from build123d import *

# Parameters (mm, degrees)
SALIENTE_EXTRUIR1_DEPTH  = 100
CROQUIS4_W               = 90
CROQUIS4_H               = 70
CORTAR_EXTRUIR1_DEPTH    = 44
SALIENTE_EXTRUIR2_DEPTH  = 19
SALIENTE_EXTRUIR4_START  = 19
SALIENTE_EXTRUIR4_DEPTH  = 19
SALIENTE_EXTRUIR7_DEPTH  = 13
SALIENTE_EXTRUIR28_START = 13
CROQUIS11_W              = 34
CROQUIS11_H              = 2.5
SALIENTE_EXTRUIR28_DEPTH = 13
CROQUIS13_W              = 28
CROQUIS13_H              = 6
SALIENTE_EXTRUIR10_DEPTH = 24
CROQUIS15_R              = 1.5
CORTAR_EXTRUIR2_DEPTH    = 5
CORTAR_EXTRUIR3_DEPTH    = 24
SALIENTE_EXTRUIR12_START = -28
SALIENTE_EXTRUIR12_DEPTH = 28
SALIENTE_EXTRUIR13_DEPTH = 52
SALIENTE_EXTRUIR14_DEPTH = 100
CORTAR_EXTRUIR4_DEPTH    = 24
SALIENTE_EXTRUIR15_DEPTH = 24
CORTAR_EXTRUIR7_DEPTH    = 90
SALIENTE_EXTRUIR27_DEPTH = 14
CORTAR_EXTRUIR12_DEPTH   = 90
CROQUIS41_R              = 2.6
CORTAR_EXTRUIR13_DEPTH   = 10
CROQUIS42_W              = 26
CROQUIS42_H              = 3.651340431
CORTAR_EXTRUIR14_DEPTH   = 121.043742028
CROQUIS37_W              = 5
CROQUIS37_H              = 25
CORTAR_EXTRUIR15_DEPTH   = 4
CROQUIS44_R              = 1.5
CORTAR_EXTRUIR16_DEPTH   = 4


with BuildPart() as part:
    # Croquis1 → Saliente-Extruir1 (new body)
    with BuildSketch(Plane(origin=(0, 0, 0), x_dir=(0, 0, -1), z_dir=(1, 0, 0))):
        with BuildLine():
            Line((50, 24), (50, 56))
            Line((50, 56), (-1.5, 56))
            Line((-1.5, 56), (-9.741455248, 56))
            ThreePointArc((-9.741455248, 56), (-16.048737738, 53.76003786), (-19.530405432, 48.043637519))
            Line((-19.530405432, 48.043637519), (-26.9291309, 12.604008733))
            Line((-26.9291309, 12.604008733), (-35.5, 0))
            Line((-35.5, 0), (-20, 0))
            Line((-20, 0), (-20, 14))
            ThreePointArc((-20, 14), (-17.071067812, 21.071067812), (-10, 24))
            Line((-10, 24), (50, 24))
        make_face()
    extrude(amount=SALIENTE_EXTRUIR1_DEPTH)

    # Croquis4 → Cortar-Extruir1 (cut, symmetric)
    with BuildSketch(Plane.XY):
        with Locations((50, 35)):
            Rectangle(CROQUIS4_W, CROQUIS4_H)
    extrude(amount=CORTAR_EXTRUIR1_DEPTH, both=True, mode=Mode.SUBTRACT)

    # Croquis5 → Saliente-Extruir2 (add)
    with BuildSketch(Plane(origin=(5, 0, 0), x_dir=(0, 0, -1), z_dir=(1, 0, 0))):
        with BuildLine():
            Line((-20, 0), (-20, 14))
            ThreePointArc((-20, 14), (-17.071067812, 21.071067812), (-10, 24))
            Line((-10, 24), (50, 24))
            Line((50, 24), (50, 26.5))
            Line((50, 26.5), (-10, 26.5))
            ThreePointArc((-10, 26.5), (-18.838834765, 22.838834765), (-22.5, 14))
            Line((-22.5, 14), (-22.5, 0))
            Line((-22.5, 0), (-20, 0))
        make_face()
    extrude(amount=SALIENTE_EXTRUIR2_DEPTH)

    # Croquis7 → Saliente-Extruir4 (add)
    with BuildSketch(Plane.ZY.offset(-95).offset(SALIENTE_EXTRUIR4_START)):
        with BuildLine():
            Line((20, 14), (20, 0))
            Line((20, 0), (22.5, 0))
            Line((22.5, 0), (22.5, 14))
            ThreePointArc((22.5, 14), (18.838834765, 22.838834765), (10, 26.5))
            Line((10, 26.5), (-50, 26.5))
            Line((-50, 26.5), (-50, 24))
            Line((-50, 24), (10, 24))
            ThreePointArc((10, 24), (17.071067812, 21.071067812), (20, 14))
        make_face()
    extrude(amount=-SALIENTE_EXTRUIR4_DEPTH)

    # Croquis10 → Saliente-Extruir7 (add)
    with BuildSketch(Plane(origin=(24, 0, 0), x_dir=(0, 0, -1), z_dir=(1, 0, 0))):
        with BuildLine():
            Line((50, 26.5), (-10, 26.5))
            ThreePointArc((-10, 26.5), (-18.838834765, 22.838834765), (-22.5, 14))
            Line((-22.5, 14), (-22.5, 0))
            Line((-22.5, 0), (-11, 0))
            Line((-11, 0), (-11, 7.2))
            ThreePointArc((-11, 7.2), (-10.121320344, 9.321320344), (-8, 10.2))
            Line((-8, 10.2), (-2, 10.2))
            ThreePointArc((-2, 10.2), (0.121320344, 9.321320344), (1, 7.2))
            Line((1, 7.2), (1, 0))
            Line((1, 0), (24, 0))
            Line((24, 0), (24, 7.2))
            ThreePointArc((24, 7.2), (24.878679656, 9.321320344), (27, 10.2))
            Line((27, 10.2), (33, 10.2))
            ThreePointArc((33, 10.2), (35.121320344, 9.321320344), (36, 7.2))
            Line((36, 7.2), (36, 0))
            Line((36, 0), (50, 0))
            Line((50, 0), (50, 26.5))
        make_face()
    extrude(amount=SALIENTE_EXTRUIR7_DEPTH)

    # Croquis11 → Saliente-Extruir28 (add)
    with BuildSketch(Plane.ZY.offset(-76).offset(SALIENTE_EXTRUIR28_START)):
        with BuildLine():
            Line((10, 24), (-10, 24))
            Line((-10, 24), (-10, 0))
            Line((-10, 0), (-1, 0))
            Line((-1, 0), (-1, 7.2))
            ThreePointArc((-1, 7.2), (-0.121320344, 9.321320344), (2, 10.2))
            Line((2, 10.2), (8, 10.2))
            ThreePointArc((8, 10.2), (10.121320344, 9.321320344), (11, 7.2))
            Line((11, 7.2), (11, 0))
            Line((11, 0), (20, 0))
            Line((20, 0), (20, 14))
            ThreePointArc((20, 14), (17.071067812, 21.071067812), (10, 24))
        make_face()
        with BuildLine():
            Line((-10, 0), (-10, 24))
            Line((-10, 24), (-44, 24))
            Line((-44, 24), (-44, 26.5))
            Line((-44, 26.5), (-50, 26.5))
            Line((-50, 26.5), (-50, 24))
            Line((-50, 24), (-50, 0))
            Line((-50, 0), (-36, 0))
            Line((-36, 0), (-36, 7.2))
            ThreePointArc((-36, 7.2), (-35.121320344, 9.321320344), (-33, 10.2))
            Line((-33, 10.2), (-27, 10.2))
            ThreePointArc((-27, 10.2), (-24.878679656, 9.321320344), (-24, 7.2))
            Line((-24, 7.2), (-24, 0))
            Line((-24, 0), (-10, 0))
        make_face()
        with Locations((-27, 25.25)):
            Rectangle(CROQUIS11_W, CROQUIS11_H)
        with BuildLine():
            Line((10, 26.5), (-10, 26.5))
            Line((-10, 26.5), (-10, 24))
            Line((-10, 24), (10, 24))
            ThreePointArc((10, 24), (17.071067812, 21.071067812), (20, 14))
            Line((20, 14), (20, 0))
            Line((20, 0), (22.5, 0))
            Line((22.5, 0), (22.5, 14))
            ThreePointArc((22.5, 14), (18.838834765, 22.838834765), (10, 26.5))
        make_face()
    extrude(amount=-SALIENTE_EXTRUIR28_DEPTH)

    # Croquis13 → Saliente-Extruir10 (add)
    with BuildSketch(Plane.XZ.offset(-24)):
        with Locations((50, -47)):
            Rectangle(CROQUIS13_W, CROQUIS13_H)
    extrude(amount=SALIENTE_EXTRUIR10_DEPTH)

    # Croquis15 → Cortar-Extruir2 (cut)
    with BuildSketch(Plane(origin=(0, 0, 0), x_dir=(1, 0, 0), z_dir=(0, 1, 0))):
        with Locations(Location((70, 38.5, 0), (0, 0, 270))):
            Circle(CROQUIS15_R)
        with Locations(Location((70, 8.5, 0), (0, 0, 270))):
            Circle(CROQUIS15_R)
        with Locations(Location((70, -18.5, 0), (0, 0, 270))):
            Circle(CROQUIS15_R)
        with Locations(Location((29, -18.5, 0), (0, 0, 90))):
            Circle(CROQUIS15_R)
        with Locations(Location((29, 8.5, 0), (0, 0, 90))):
            Circle(CROQUIS15_R)
        with Locations(Location((29, 38.5, 0), (0, 0, 90))):
            Circle(CROQUIS15_R)
    extrude(amount=CORTAR_EXTRUIR2_DEPTH, mode=Mode.SUBTRACT)

    # Croquis16 → Cortar-Extruir3 (cut)
    with BuildSketch(Plane(origin=(100, 0, 0), x_dir=(0, 0, -1), z_dir=(1, 0, 0))):
        with BuildLine():
            Line((10, 24.25), (10, 24))
            Line((10, 24), (50, 24))
            Line((50, 24), (50.733673202, 24))
            Line((50.733673202, 24), (50.733673202, 28.25))
            Line((50.733673202, 28.25), (50, 28.25))
            Line((50, 28.25), (50, 27.25))
            ThreePointArc((50, 27.25), (49.414213562, 25.835786438), (48, 25.25))
            Line((48, 25.25), (11, 25.25))
            Line((11, 25.25), (10, 25.25))
            Line((10, 25.25), (10, 24.25))
        make_face()
    extrude(amount=-CORTAR_EXTRUIR3_DEPTH, mode=Mode.SUBTRACT)

    # Croquis17 → Saliente-Extruir12 (add)
    with BuildSketch(Plane(origin=(100, 0, 0), x_dir=(0, 0, -1), z_dir=(1, 0, 0)).offset(SALIENTE_EXTRUIR12_START)):
        with BuildLine():
            Line((-14, 20.944171176), (7, 20.944171176))
            Line((7, 20.944171176), (10, 20.944171176))
            Line((10, 20.944171176), (10, 23.944171176))
            Line((10, 23.944171176), (10, 24))
            Line((10, 24), (10, 26.5))
            Line((10, 26.5), (-10, 26.5))
            ThreePointArc((-10, 26.5), (-18.838834765, 22.838834765), (-22.5, 14))
            Line((-22.5, 14), (-20, 14))
            Line((-20, 14), (-20, 14.944171176))
            ThreePointArc((-20, 14.944171176), (-18.242640687, 19.186811864), (-14, 20.944171176))
        make_face()
    extrude(amount=SALIENTE_EXTRUIR12_DEPTH)

    # Croquis18 → Saliente-Extruir13 (add)
    with BuildSketch(Plane(origin=(76, 0, 0), x_dir=(0, 0, -1), z_dir=(1, 0, 0))):
        Polygon((50, 0), (50, 56), (59.5, 56), align=None)
    extrude(amount=-SALIENTE_EXTRUIR13_DEPTH)

    # Croquis19 → Saliente-Extruir14 (add)
    with BuildSketch(Plane(origin=(100, 0, 0), x_dir=(0, 0, -1), z_dir=(1, 0, 0))):
        with BuildLine():
            Line((48, 25.25), (54.283482143, 25.25))
            Line((54.283482143, 25.25), (59.5, 56))
            Line((59.5, 56), (50, 56))
            Line((50, 56), (50, 27.25))
            ThreePointArc((50, 27.25), (49.414213562, 25.835786438), (48, 25.25))
        make_face()
    extrude(amount=-SALIENTE_EXTRUIR14_DEPTH)

    # Croquis20 → Cortar-Extruir4 (cut)
    with BuildSketch(Plane.ZY):
        Polygon((-48, 25.25), (-50.733673202, 25.25), (-50.733673202, 24), (-50, 24), (-10, 24), (-10, 24.25), (-10, 25.25), (-11, 25.25), align=None)
    extrude(amount=-CORTAR_EXTRUIR4_DEPTH, mode=Mode.SUBTRACT)

    # Croquis21 → Saliente-Extruir15 (add)
    with BuildSketch(Plane.ZY):
        with BuildLine():
            Line((20, 14.944171176), (20, 14))
            Line((20, 14), (22.5, 14))
            ThreePointArc((22.5, 14), (18.838834765, 22.838834765), (10, 26.5))
            Line((10, 26.5), (-10, 26.5))
            Line((-10, 26.5), (-10, 24))
            Line((-10, 24), (-10, 23.944171176))
            Line((-10, 23.944171176), (-10, 20.944171176))
            Line((-10, 20.944171176), (-7, 20.944171176))
            Line((-7, 20.944171176), (14, 20.944171176))
            ThreePointArc((14, 20.944171176), (18.242640687, 19.186811864), (20, 14.944171176))
        make_face()
    extrude(amount=-SALIENTE_EXTRUIR15_DEPTH)

    # Croquis23 → Cortar-Extruir7 (cut)
    with BuildSketch(Plane(origin=(5, 0, 0), x_dir=(0, 0, -1), z_dir=(1, 0, 0))):
        Polygon((44, 56), (53.5, 56), (47.651340431, 26.5), (44, 26.5), align=None)
    extrude(amount=CORTAR_EXTRUIR7_DEPTH, mode=Mode.SUBTRACT)

    # Croquis39 → Saliente-Extruir27 (add)
    with BuildSketch(Plane(origin=(0, 0, 0), x_dir=(1, 0, 0), z_dir=(0, 1, 0))):
        Polygon((5, -26.5), (5, -35.5), (95, -35.5), (95, -26.5), (95, -22.5), (5, -22.5), align=None)
    extrude(amount=SALIENTE_EXTRUIR27_DEPTH)

    # Croquis40 → Cortar-Extruir12 (cut)
    with BuildSketch(Plane(origin=(95, 0, 0), x_dir=(0, 0, -1), z_dir=(1, 0, 0))):
        Polygon((-26.637690033, 14), (-35.5, 14), (-35.5, 0), (-26.9291309, 12.604008733), align=None)
    extrude(amount=-CORTAR_EXTRUIR12_DEPTH, mode=Mode.SUBTRACT)

    # Croquis41 → Cortar-Extruir13 (cut)
    with BuildSketch(Plane(origin=(0, -8.087799177, -40.793975597), x_dir=(1, 0, 0), z_dir=(0, 0.19447439298800823, 0.9809075952769181))):
        with Locations(Location((50, 58.257848261, 0), (0, 0, 270))):
            Circle(CROQUIS41_R)
    extrude(amount=-CORTAR_EXTRUIR13_DEPTH, mode=Mode.SUBTRACT)

    # Croquis42 → Cortar-Extruir14 (cut, through all)
    with BuildSketch(Plane(origin=(0, 26.5, 0), x_dir=(1, 0, 0), z_dir=(0, 1, 0))):
        with Locations((50, 45.825670215)):
            Rectangle(CROQUIS42_W, CROQUIS42_H)
    extrude(amount=-CORTAR_EXTRUIR14_DEPTH, mode=Mode.SUBTRACT)

    # Croquis37 → Cortar-Extruir15 (cut)
    with BuildSketch(Plane(origin=(0, 56, 0), x_dir=(1, 0, 0), z_dir=(0, 1, 0))):
        with Locations((97.5, 27)):
            Rectangle(CROQUIS37_W, CROQUIS37_H)
        with Locations((2.5, 27)):
            Rectangle(CROQUIS37_W, CROQUIS37_H)
    extrude(amount=-CORTAR_EXTRUIR15_DEPTH, mode=Mode.SUBTRACT)

    # Croquis44 → Cortar-Extruir16 (cut)
    with BuildSketch(Plane.XZ):
        with Locations(Location((50, 33.5, 0), (0, 0, 270))):
            Circle(CROQUIS44_R)
        with Locations(Location((33.5, 33.5, 0), (0, 0, 270))):
            Circle(CROQUIS44_R)
        with Locations(Location((16.5, 33.5, 0), (0, 0, 270))):
            Circle(CROQUIS44_R)
        with Locations(Location((83.5, 33.5, 0), (0, 0, 331.312619738))):
            Circle(CROQUIS44_R)
        with Locations(Location((66.5, 33.5, 0), (0, 0, 331.312619738))):
            Circle(CROQUIS44_R)
    extrude(amount=-CORTAR_EXTRUIR16_DEPTH, mode=Mode.SUBTRACT)


solid = part.part
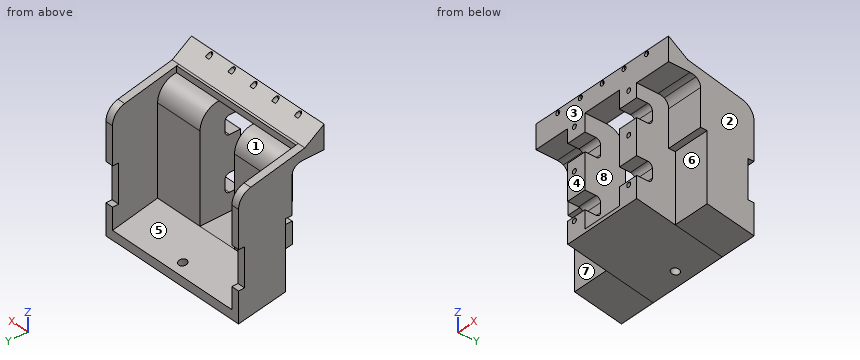
Work out the finished part from the listing and answer in its coordinate system (mm). Face numbers are marked on the shaded views. A direction names the side the tool comes from. Coordinates: 2 decimals unless noted, no trailing zeros. Loops run counter-clockwise (first coordinate to the right, second up) from the corner with the lowest first, then second, coordinate; pieces in that order, holes last. Notation, with made-up numbers: (6.5, 56.25) -> (15.5, 56.25) arc R10 cw to (15.5, 66.25) -> close; hole circle Ø3 at (30, 66.25). An arc over 180 degrees is marked (long way). Write each question's results on one line, items separated by ' | '. Start each with the question number.
1) Find section B-B on x = 45. Determine the outline of the cut face in (y, z), then the cut area to 3 significant figures.
2) Find section A-A on z = -8.5. Determine the outline of the cut face in (x, y).
3) Consider line 1 along X through (y, z) = (1.2, 33.5); line 2 along X through (y, z) = (1.9, -8.5); line 3 along X through (y, z) = (22.5, 5). Determine where each line is inside the solid, lowest interval first.
4) The mould has two halves that part along X. Classify the marked faces 1, 2 and 3: pulls with the +X half, pulls with the -X half, needs draft (parallel to the pull), parting line crosses it, or undercut.
5) For the marked faces 4, 5, 6, 7 and 8, determine the directions among +Z, -Z, +X, -X, +Y, -Y from which every point of the face is accessible in a straight line to the end or side of a thin tool.
6) Find section C-C on x = 8.5. Determine the outline of the cut face in (y, z), then the cut area to 3 significant figures.
7) Flat-ended cylindrical pins translate along their axes: P1, Ø2.5, axis at x = 29, z = -8.5, coming from the +Y side; P2, Ø8, axis at x = 71, z = -24, coming from the -Y side; P3, Ø1, axis at x = 28.5, y = 50, coming from the +Z side; P4, Ø1.8, axis at x = 70, z = -8.5, coming from the -Y side. Find the tip coordinate at first contact, or state that the pin passes through.
8) Find section D-D on z = -21. Determine the outline of the cut face in (x, y), then the cut area to 3 significant figures.
Response values:
1) outline: (0, -50) -> (56, -59.5) -> (56, -53.5) -> (26.5, -47.65) -> (0, -47.65) -> close; (0, 22.5) -> (14, 22.5) -> (14, 26.64) -> (12.6, 26.93) -> (0, 35.5) -> close | area: 427 mm^2
2) outline: (0, 20.94) -> (24, 20.94) -> (24, 0) -> (27.5, 0) -> (27.5, 5) -> (30.5, 5) -> (30.5, 0) -> (37, 0) -> (37, 26.5) -> (5, 26.5) -> (5, 56) -> (0, 56) -> close; (63, 0) -> (68.5, 0) -> (68.5, 5) -> (71.5, 5) -> (71.5, 0) -> (76, 0) -> (76, 20.94) -> (100, 20.94) -> (100, 56) -> (95, 56) -> (95, 26.5) -> (63, 26.5) -> close
3) line 1: x = 0 to 15, 18 to 32, 35 to 48.5, 51.5 to 65, 68 to 82, 85 to 100 | line 2: x = 24 to 27.5, 30.5 to 37, 63 to 68.5, 71.5 to 76 | line 3: x = 0 to 37, 63 to 100
4) face 1: undercut | face 2: pulls with the +X half | face 3: needs draft
5) face 4: +Z, -Z, +X, -X, -Y | face 5: +Z, +Y | face 6: -Z, +X, -Y | face 7: -Z, -X, -Y | face 8: +Y, -Y
6) outline: (0, 20) -> (14, 20) arc R10 cw to (17.99, 19.17) arc R6 cw to (20.94, 14) -> (20.94, -10) -> (25.25, -10) -> (25.25, -54.28) -> (56, -59.5) -> (56, -53.5) -> (26.5, -47.65) -> (26.5, 10) arc R12.5 ccw to (14, 22.5) -> (14, 26.64) -> (12.6, 26.93) -> (0, 35.5) -> close | area: 568 mm^2
7) P1: stops at y = 26.5 | P2: stops at y = 0 | P3: stops at z = -52.21 | P4: stops at y = 5
8) outline: (0, 25.25) -> (24, 25.25) -> (24, 0) -> (37, 0) -> (37, 26.5) -> (5, 26.5) -> (5, 52) -> (0, 52) -> close; (63, 0) -> (76, 0) -> (76, 25.25) -> (100, 25.25) -> (100, 52) -> (95, 52) -> (95, 26.5) -> (63, 26.5) -> close | area: 1,000 mm^2
